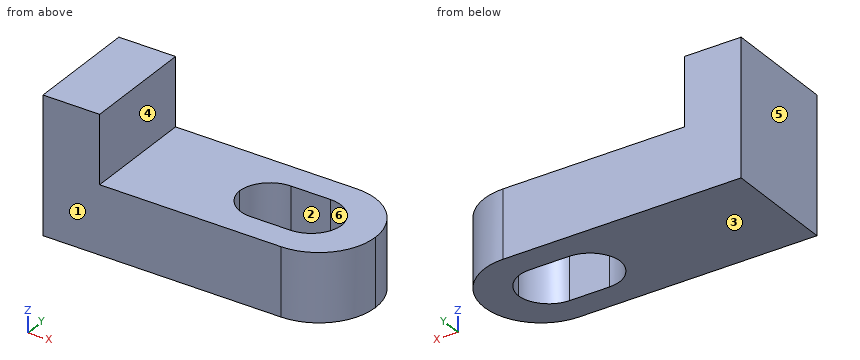
from build123d import *

# Parameters (mm, degrees)
F0_W        = 21
F0_H        = 10
F0_W_2      = 9
F0_H_2      = 5.3
F0_W_3      = 5
F1_DEPTH    = 6
F2_DEPTH    = 12
F3_T1_DEPTH = 6
F4_R        = 4.99999


# Not quite as in the source:
# - a fillet or chamfer that OpenCascade refuses, or shapes differently, is made with other operations: its cross-section is extruded or revolved along the edge and cut away or added
# - a fillet or chamfer is up to 0.001 mm smaller than in the source, because OpenCascade refuses the exact size


with BuildPart() as f1:
    # F0 (on Top) → F1 (new body)
    with BuildSketch(Plane.XY):
        with Locations((-10.5, 5)):
            Rectangle(F0_W, F0_H)
        with Locations((-7.5, 5)):
            Rectangle(F0_W_2, F0_H_2, mode=Mode.SUBTRACT)
        with Locations((-23.5, 5)):
            Rectangle(F0_W_3, F0_H)
    extrude(amount=F1_DEPTH)

    # F0 (on Top) → F2 (join)
    with BuildSketch(Plane.XY):
        with Locations((-23.5, 5)):
            Rectangle(F0_W_3, F0_H)
    extrude(amount=F2_DEPTH)

    # F3: fillet of radius 2.75 on 4 edges, made by hand

    # F3_s2 → F3_t1 (join)
    with BuildSketch(Plane.XY):
        with BuildLine():
            ThreePointArc((-9.25, 7.65), (-11.1945436483, 6.8445436483), (-12, 4.9))
            Line((-12, 4.9), (-12, 7.65))
            Line((-12, 7.65), (-9.25, 7.65))
        make_face()
        with BuildLine():
            ThreePointArc((-12, 5.1), (-11.1945436483, 3.1554563517), (-9.25, 2.35))
            Line((-9.25, 2.35), (-12, 2.35))
            Line((-12, 2.35), (-12, 5.1))
        make_face()
        with BuildLine():
            ThreePointArc((-5.75, 7.65), (-3.8054563517, 6.8445436483), (-3, 4.9))
            Line((-3, 4.9), (-3, 7.65))
            Line((-3, 7.65), (-5.75, 7.65))
        make_face()
        with BuildLine():
            ThreePointArc((-3, 5.1), (-3.8054563517, 3.1554563517), (-5.75, 2.35))
            Line((-5.75, 2.35), (-3, 2.35))
            Line((-3, 2.35), (-3, 5.1))
        make_face()
    extrude(amount=F3_T1_DEPTH)

    # F4 (radius 5 in the source; OpenCascade refuses exactly that, so slightly less here)
    f4_edges = [f1.edges().sort_by_distance(p)[0] for p in [
        (0, 0, 3),
        (0, 10, 3),
    ]]
    fillet(f4_edges, radius=F4_R)


solid = f1.part
CAD build for the part. Positions are in the model's coordinates, mm. Face numbers are marked on the shaded views. A direction names the side the tool comes from. Coordinates: 2 decimals unless noted, no trailing zeros. Order: outer loops, then holes, each group sorted by start corner. A loop starts at its lowest first (then second) coordinate and runs counter-clockwise, first axis right, second up.
Item 1: Band-saw the part on C-C on x = -10.75. List the corners of the cut face in (y, z).
Check sheet entries:
outline: (0, 0) - (2.8, 0) - (2.8, 6) - (0, 6) - close; (7.2, 0) - (10, 0) - (10, 6) - (7.2, 6) - close
Item 2: 3-axis set-ups, long thin cutter, end or side, ignore diameter. For the marked faces 4, 5 and 6: which of +Z, -Z, +X, -X, +Y, -Y reach the whole face in a straight line?
Check sheet entries:
face 4: +Z, +X, +Y, -Y
face 5: +Z, -Z, -X, +Y, -Y
face 6: +Z, -Z
Item 3: Two-plate mould, pull along Y, no slides. Class the marked faces 1, 2 and 3: +Y half, -Y half, draft (parallel to the pull), parting line (faces both ways), or undercut.
Check sheet entries:
face 1: -Y half
face 2: undercut
face 3: draft
Item 4: Pin check, flat tips, straight feed: pin 1 Ø4 at (x, y) = (-6.5, 1.5) entering from +Z; pin 2 Ø6 at (y, z) = (1.5, 5.5) entering from +X; pin 3 Ø1.8 at (y, z) = (5, 9) entering from +X. Stop position of each tip, or through.
Check sheet entries:
pin 1: stops at z = 6
pin 2: stops at x = -0.03
pin 3: stops at x = -21
Item 5: Drill centre lines: L1, parallel to Y at x = -6.75, z = 5.5; L2, parallel to Z at x = -17.75, y = 4; L3, parallel to X at y = 8.5, z = 8.75. Where is each one in solid material? Low to high.
Check sheet entries:
L1: y = 0 to 2.35, 7.65 to 10
L2: z = 0 to 6
L3: x = -26 to -21
Item 6: Band-saw the part on A-A on y = 6. List the corners of the cut face in (x, z).
Check sheet entries:
outline: (-26, 0) - (-11.77, 0) - (-11.77, 6) - (-21, 6) - (-21, 12) - (-26, 12) - close; (-3.23, 0) - (-0.1, 0) - (-0.1, 6) - (-3.23, 6) - close
Item 7: Band-saw the part on D-D on y = 2. List the corners of the cut face in (x, z).
Check sheet entries:
outline: (-26, 0) - (-1, 0) - (-1, 6) - (-21, 6) - (-21, 12) - (-26, 12) - close
